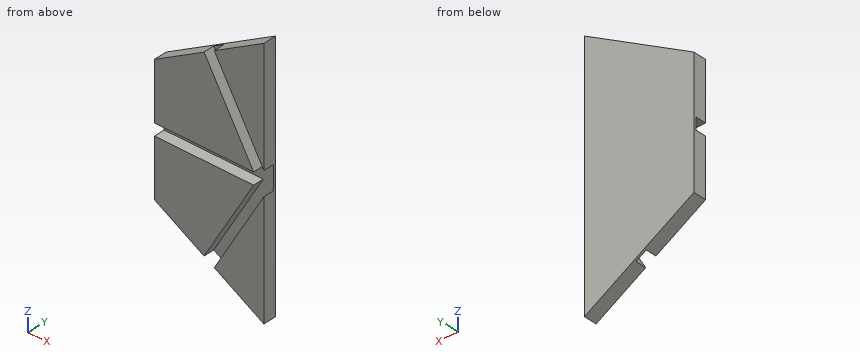
from build123d import *

# Parameters (mm, degrees)
BOSS_EXTRUDE1_DEPTH     = 6
SKETCH2_W               = 100
SKETCH2_H               = 5.4
CUT_EXTRUDE_THIN1_DEPTH = 5
INTERSECT1_DEPTH        = 50


# Read off the part's stored shape, not the designer's step: Intersect1
with BuildPart() as part:
    # Sketch1 → Boss-Extrude1 (new body)
    with BuildSketch(Plane(origin=(0, 0, 0), x_dir=(1, 0, 0), z_dir=(0, 1, 0))):
        Polygon((0, 57.735026919), (-50, 28.867513459), (-50, -28.867513459), (0, -57.735026919), (50, -28.867513459), (50, 28.867513459), align=None)
    extrude(amount=BOSS_EXTRUDE1_DEPTH)

    # Sketch2 → Cut-Extrude-Thin1 (cut)
    with BuildSketch(Plane.XZ):
        Polygon((-27.33826859, 41.951270189), (22.66173141, -44.651270189), (27.33826859, -41.951270189), (-22.66173141, 44.651270189), align=None)
        Polygon((22.66173141, 44.651270189), (-27.33826859, -41.951270189), (-22.66173141, -44.651270189), (27.33826859, 41.951270189), align=None)
        Rectangle(SKETCH2_W, SKETCH2_H)
    extrude(amount=-CUT_EXTRUDE_THIN1_DEPTH, mode=Mode.SUBTRACT)

    # Intersect1 outline → Intersect1 (cut)
    with BuildSketch(Plane.YZ):
        Polygon((0, 2.7), (5, 2.7), (5, -2.7), (0, -2.7), (0, -59), (6, -59), (6, 59), (0, 59), align=None)
    extrude(amount=INTERSECT1_DEPTH, mode=Mode.SUBTRACT)


solid = part.part
Geometry: final body of the model. Coordinates: model frame, mm. Give positions to 0.01 mm unless a question says otherwise; leave off trailing zeros. Write each loop counter-clockwise with the first axis right and the second up, starting at its lowest first coordinate (ties: lowest second). Pieces come first, ordered by that corner, then holes. Notation, with made-up numbers: (16, -9.75) -> (30, -9.75) arc R32 ccw to (30, 24.25) -> close; hole circle Ø6 at (5.25, -30.5). An arc over 180 degrees is marked (long way). Answer in a Markdown table with one row per item.
(1) Section query C-C on z = -31.5. Return loops of the section in (x, y), then the cut area to 3 significant figures.
Answers below:
| item | result |
|---|---|
| outline | (-45.44, 0) -> (-21.3, 0) -> (-21.3, 5) -> (-15.07, 5) -> (-15.07, 0) -> (0, 0) -> (0, 6) -> (-45.44, 6) -> close |
| area | 241 mm^2 |
(2) Section query A-A on y = 3.3. Return loops of the section in (x, z), then the cut area to 3 significant figures.
Answers below:
| item | result |
|---|---|
| outline | (-50, -28.87) -> (-27.34, -41.95) -> (-4.68, -2.7) -> (-50, -2.7) -> close; (-50, 2.7) -> (-4.68, 2.7) -> (-27.34, 41.95) -> (-50, 28.87) -> close; (-22.66, -44.65) -> (0, -57.74) -> (0, -5.4) -> close; (-22.66, 44.65) -> (0, 5.4) -> (0, 57.74) -> close |
| area | 3,560 mm^2 |
(3) Section query B-B on x = -7. Return loops of the section in (y, z), then the cut area to 3 significant figures.
Answers below:
| item | result |
|---|---|
| outline | (0, -53.69) -> (6, -53.69) -> (6, 53.69) -> (0, 53.69) -> (0, 17.52) -> (5, 17.52) -> (5, 6.72) -> (0, 6.72) -> (0, 2.7) -> (5, 2.7) -> (5, -2.7) -> (0, -2.7) -> (0, -6.72) -> (5, -6.72) -> (5, -17.52) -> (0, -17.52) -> close |
| area | 509 mm^2 |
(4) Ray query, line 1 along Z through (x, y) = (-22, 3.4); line 2 along Z through (x, y) = (-9, 2.7); line 3 along Z through (x, y) = (-47.5, 3.6). Return the intervals inside material, ascending. Write a range as [from, to].
Answers below:
| item | result |
|---|---|
| line 1 | [-45.03, -43.51], [-32.71, -2.7], [2.7, 32.71], [43.51, 45.03] |
| line 2 | [-52.54, -20.99], [-10.19, -2.7], [2.7, 10.19], [20.99, 52.54] |
| line 3 | [-30.31, -2.7], [2.7, 30.31] |
(5) Section query D-D on x = -12.5. Return loops of the section in (y, z).
Answers below:
| item | result |
|---|---|
| outline | (0, -50.52) -> (6, -50.52) -> (6, 50.52) -> (0, 50.52) -> (0, 27.05) -> (5, 27.05) -> (5, 16.25) -> (0, 16.25) -> (0, 2.7) -> (5, 2.7) -> (5, -2.7) -> (0, -2.7) -> (0, -16.25) -> (5, -16.25) -> (5, -27.05) -> (0, -27.05) -> close |
(6) Pin query (flat end, axial travel): pin 1 (3 mm diameter, centred on x = -37, z = -29, fed in from -Y); pin 2 (1 mm diameter, centred on y = 3, z = 42.5, fed in from -X); pin 3 (2 mm diameter, centred on x = -5.5, y = 4.5, fed in from -Z); pin 4 (1.5 mm diameter, centred on x = -34.5, y = 2.5, fed in from -Z). Return the tip coordinate at first contact, or that it passes through.
Answers below:
| item | result |
|---|---|
| pin 1 | y = 0 |
| pin 2 | x = -21.71 |
| pin 3 | z = -55.14 |
| pin 4 | z = -38.25 |
